Work out the finished part from the listing and answer in its coordinate system (mm). Face numbers are marked on the shaded views. Round coordinates to 2 decimals unless told otherwise and drop trailing zeros. Order: outer loops, then holes, each group sorted by start corner. A loop starts at its lowest first (then second) coordinate and runs counter-clockwise, first axis right, second up. Notation, with made-up numbers: (73.5, -9.5) - (102.5, -9.5) arc R14 cw to (102.5, 8.5) - close; hole circle Ø10 at (41, -36.75). An arc over 180 degrees is marked (long way). Answer in a Markdown table with one row per item.
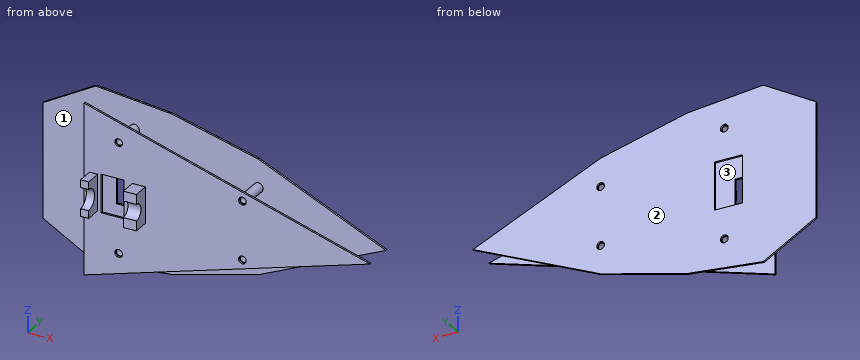
from build123d import *

# Parameters (mm, degrees)
STOCK_BODY2_2_1_START         = -47.04864598
STOCK_BODY2_2_1_OUTLINE_W     = 43.787012176
STOCK_BODY2_2_1_OUTLINE_H     = 74.629705784
STOCK_BODY2_2_1_OUTLINE_R     = 6
STOCK_BODY2_2_1_DEPTH         = 3
STOCK_BODY2_2_1_START_2       = -92.04864598
STOCK_BODY2_2_1_2_OUTLINE_R   = 6
STOCK_BODY2_2_1_2_OUTLINE_W   = 35.905709945
STOCK_BODY2_2_1_2_OUTLINE_H   = 59.945220798
STOCK_BODY2_2_1_2_DEPTH       = 3
STOCK_BODY2_2_1_START_3       = -89.04864598
STOCK_BODY2_2_1_3_OUTLINE_R   = 7.5
STOCK_BODY2_2_1_3_OUTLINE_R_2 = 5
STOCK_BODY2_2_1_3_DEPTH       = 42
SCALE1_SCALE                  = 1.5
SKETCH2_W                     = 19.240593306
SKETCH2_H                     = 84.91603611
BOSS_EXTRUDE1_DEPTH           = 38.1
SKETCH3_W                     = 30.633251364
SKETCH3_H                     = 84.659976372
BOSS_EXTRUDE2_DEPTH           = 38.1
SKETCH4_R                     = 19.304
CUT_EXTRUDE2_DEPTH            = 31.6738
SKETCH5_R                     = 24.765
CUT_EXTRUDE3_DEPTH            = 31.6738


# Read off the part's stored shape, not the designer's step: Stock-Body2.2-1
with BuildPart() as part:
    # Stock-Body2.2-1 outline → Stock-Body2.2-1 (new body)
    with BuildSketch(Plane(origin=(0, 0, 0), x_dir=(1, 0, 0), z_dir=(0, 1, 0)).offset(STOCK_BODY2_2_1_START)):
        Polygon((135.362738013, -89.648548647), (334.939803936, 0), (135.362738013, 89.648548647), (0, 124.445224737), (-119.088720056, 136.857824586), (-201.515305017, 89.648548647), (-201.515305017, -89.648548647), (-119.088720056, -136.857824586), (0, -124.445224737), align=None)
        with Locations((-64.591790786, 0)):
            Rectangle(STOCK_BODY2_2_1_OUTLINE_W, STOCK_BODY2_2_1_OUTLINE_H, mode=Mode.SUBTRACT)
        with Locations((-58.24622251, -85.855051723)):
            Circle(STOCK_BODY2_2_1_OUTLINE_R, mode=Mode.SUBTRACT)
        with Locations((135.362738013, -45.618949287)):
            Circle(STOCK_BODY2_2_1_OUTLINE_R, mode=Mode.SUBTRACT)
        with Locations((-58.24622251, 85.855051723)):
            Circle(STOCK_BODY2_2_1_OUTLINE_R, mode=Mode.SUBTRACT)
        with Locations((135.362738013, 45.618949287)):
            Circle(STOCK_BODY2_2_1_OUTLINE_R, mode=Mode.SUBTRACT)
    extrude(amount=STOCK_BODY2_2_1_DEPTH)



with BuildPart() as body_2:
    # Stock-Body2.2-1 2 outline → Stock-Body2.2-1 2 (new body)
    with BuildSketch(Plane(origin=(0, 0, 0), x_dir=(1, 0, 0), z_dir=(0, 1, 0)).offset(STOCK_BODY2_2_1_START_2)):
        Polygon((-112.290148162, -133.312365233), (334.939803936, 0), (-112.290148162, 133.312365233), align=None)
        with Locations((-58.24622251, -85.855051723)):
            Circle(STOCK_BODY2_2_1_2_OUTLINE_R, mode=Mode.SUBTRACT)
        with Locations((135.362738013, -45.618949287)):
            Circle(STOCK_BODY2_2_1_2_OUTLINE_R, mode=Mode.SUBTRACT)
        with Locations((-67.509316896, 0)):
            Rectangle(STOCK_BODY2_2_1_2_OUTLINE_W, STOCK_BODY2_2_1_2_OUTLINE_H, mode=Mode.SUBTRACT)
        with Locations((-58.24622251, 85.855051723)):
            Circle(STOCK_BODY2_2_1_2_OUTLINE_R, mode=Mode.SUBTRACT)
        with Locations((135.362738013, 45.618949287)):
            Circle(STOCK_BODY2_2_1_2_OUTLINE_R, mode=Mode.SUBTRACT)
    extrude(amount=STOCK_BODY2_2_1_2_DEPTH)


with BuildPart() as part_1:
    add(part.part)

    add(body_2.part)  # Stock-Body2.2-1 3 merges body 2
    # Stock-Body2.2-1 3 outline → Stock-Body2.2-1 3 (add)
    # profile 1 of 4: a face of its own
    with BuildSketch(Plane(origin=(0, 0, 0), x_dir=(1, 0, 0), z_dir=(0, 1, 0)).offset(STOCK_BODY2_2_1_START_3)):
        with Locations((135.362738013, -45.618949287)):
            Circle(STOCK_BODY2_2_1_3_OUTLINE_R)
        with Locations((135.362738013, -45.618949287)):
            Circle(STOCK_BODY2_2_1_3_OUTLINE_R_2, mode=Mode.SUBTRACT)
    # profile 2 of 4: a face of its own
    with BuildSketch(Plane(origin=(0, 0, 0), x_dir=(1, 0, 0), z_dir=(0, 1, 0)).offset(STOCK_BODY2_2_1_START_3)):
        with Locations((-58.24622251, 85.855051723)):
            Circle(STOCK_BODY2_2_1_3_OUTLINE_R)
        with Locations((-58.24622251, 85.855051723)):
            Circle(STOCK_BODY2_2_1_3_OUTLINE_R_2, mode=Mode.SUBTRACT)
    # profile 3 of 4: a face of its own
    with BuildSketch(Plane(origin=(0, 0, 0), x_dir=(1, 0, 0), z_dir=(0, 1, 0)).offset(STOCK_BODY2_2_1_START_3)):
        with Locations((135.362738013, 45.618949287)):
            Circle(STOCK_BODY2_2_1_3_OUTLINE_R)
        with Locations((135.362738013, 45.618949287)):
            Circle(STOCK_BODY2_2_1_3_OUTLINE_R_2, mode=Mode.SUBTRACT)
    # profile 4 of 4: a face of its own
    with BuildSketch(Plane(origin=(0, 0, 0), x_dir=(1, 0, 0), z_dir=(0, 1, 0)).offset(STOCK_BODY2_2_1_START_3)):
        with Locations((-58.24622251, -85.855051723)):
            Circle(STOCK_BODY2_2_1_3_OUTLINE_R)
        with Locations((-58.24622251, -85.855051723)):
            Circle(STOCK_BODY2_2_1_3_OUTLINE_R_2, mode=Mode.SUBTRACT)
    extrude(amount=STOCK_BODY2_2_1_3_DEPTH)


with BuildPart() as part_2:
    # Scale1: scaled about (21.693705028, -62.849152598, 0)
    add(part_1.part.scale(SCALE1_SCALE).moved(Location((-10.846852514, 31.424576299, 0))))

    # Sketch2 → Boss-Extrude1 (add)
    with BuildSketch(Plane.XZ.offset(106.648392671)):
        with Locations((-156.897972987, 0)):
            Rectangle(SKETCH2_W, SKETCH2_H)
    extrude(amount=BOSS_EXTRUDE1_DEPTH)

    # Sketch3 → Boss-Extrude2 (add)
    with BuildSketch(Plane.XZ.offset(106.648392671)):
        with Locations((-50.580967258, 0)):
            Rectangle(SKETCH3_W, SKETCH3_H)
    extrude(amount=BOSS_EXTRUDE2_DEPTH)

    # Sketch4 → Cut-Extrude2 (cut)
    with BuildSketch(Plane(origin=(-35.264341576, 0, 0), x_dir=(0, 0, -1), z_dir=(1, 0, 0))):
        with Locations((0, -144.748392671)):
            Circle(SKETCH4_R)
    extrude(amount=-CUT_EXTRUDE2_DEPTH, mode=Mode.SUBTRACT)

    # Sketch5 → Cut-Extrude3 (cut)
    with BuildSketch(Plane.ZY.offset(166.51826964)):
        with Locations((0, -144.748392671)):
            Circle(SKETCH5_R)
    extrude(amount=-CUT_EXTRUDE3_DEPTH, mode=Mode.SUBTRACT)


solid = part_2.part
1) Find section B-B, the plane y = -90.5. Give the vertices of the cut face in (x, z), then the cut area to 3 significant figures.
Filled in:
| item | result |
|---|---|
| outline | circle Ø22.5 at (-98.22, -128.78); circle Ø22.5 at (-98.22, 128.78); circle Ø22.5 at (192.2, -68.43); circle Ø22.5 at (192.2, 68.43); hole circle Ø15 at (-98.22, -128.78); hole circle Ø15 at (-98.22, 128.78); hole circle Ø15 at (192.2, -68.43); hole circle Ø15 at (192.2, 68.43) |
| area | 884 mm^2 |
2) Find section A-A, the plane x = 238. Give the vertices of the cut face in (y, z), then the cut area to 3 significant figures.
Filled in:
| item | result |
|---|---|
| outline | (-106.65, -75.58) - (-102.15, -75.58) - (-102.15, 75.58) - (-106.65, 75.58) - close; (-39.15, -113.9) - (-34.65, -113.9) - (-34.65, 113.9) - (-39.15, 113.9) - close |
| area | 1,710 mm^2 |
3) Each of these flat-tipped pins is pushed along its axis until it touches: pin 1 (11 mm diameter, centred on x = -98.22, z = -128.78, fed in from -Y); pin 2 (15.5 mm diameter, centred on x = -152.5, y = -133.5, fed in from -Z); pin 3 (4 mm diameter, centred on x = 367.5, z = -39, fed in from -Y); pin 4 (2 mm diameter, centred on y = -105.5, z = -2.5, fed in from -X). Where does it stop, or does it pass through?
Filled in:
| item | result |
|---|---|
| pin 1 | passes through |
| pin 2 | stops at z = -42.46 |
| pin 3 | stops at y = -106.65 |
| pin 4 | stops at x = -179.28 |
4) Find the intervals of material crossed by probe 1 along Y at (x, z) = (-97.5, -90); probe 2 along Y at (x, z) = (-250, -152.5); probe 3 along X at (y, z) = (-95.5, -60), in increasing order. Write a range as from..to.
Filled in:
| item | result |
|---|---|
| probe 1 | y = -106.65..-102.15, -39.15..-34.65 |
| probe 2 | y = -39.15..-34.65 |
| probe 3 | x = 184.75..199.65 |
5) Find section C-C, the plane z = -152. Give the vertices of the cut face in (x, y), then the cut area to 3 significant figures.
Filled in:
| item | result |
|---|---|
| outline | (-282.52, -39.15) - (124.01, -39.15) - (124.01, -34.65) - (-282.52, -34.65) - close; (-179.28, -106.65) - (-18.36, -106.65) - (-18.36, -102.15) - (-179.28, -102.15) - close |
| area | 2,550 mm^2 |
6) The mould has two halves that part along Y. Classify the marked faces 1, 2 and 3: released by +Y, released by -Y, zero draft, split by the parting line, or undercut.
Filled in:
| item | result |
|---|---|
| face 1 | undercut |
| face 2 | released by +Y |
| face 3 | undercut |
7) Find section D-D, the plane x = -211.5. Give the vertices of the cut face in (y, z).
Filled in:
| item | result |
|---|---|
| outline | (-39.15, -192.67) - (-34.65, -192.67) - (-34.65, 192.67) - (-39.15, 192.67) - close |
